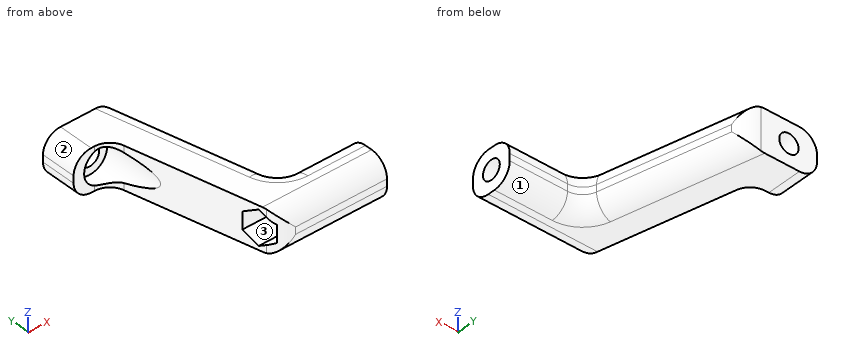
```python
from build123d import *

# Parameters (mm, degrees)
F1_DEPTH     = 12
F3_START     = -10
F2_R         = 2.75
F3_DEPTH     = 40.001
F4_DEPTH     = 50.001
F5_R         = 2.75
F6_DEPTH     = 55.001
F7_START     = -6
F5_R_2       = 5
F7_DEPTH     = 49.001
F8_T1_DEPTH  = 12
F8_T6_DEPTH  = 11.4445693846
F8_S7_R      = 5
F8_T8_DEPTH  = 8
F8_T12_DEPTH = 11.4445693846
F8_S13_R     = 5
F8_T14_DEPTH = 8
F8_T15_DEPTH = 55
F8_T17_DEPTH = 35
F8_T19_DEPTH = 28.9335864126
F8_T21_DEPTH = 32.0542901591
F8_T23_DEPTH = 52.5380765975
F8_T26_ANGLE = 77.4711922908
F8_T28_ANGLE = 77.4711922908


# Not quite as in the source:
# - a fillet or chamfer that OpenCascade refuses, or shapes differently, is made with other operations: its cross-section is extruded or revolved along the edge and cut away or added


with BuildPart() as f1:
    # F0 (on Top) → F1 (new body)
    with BuildSketch(Plane.XY):
        Polygon((-5.2704296331, 25.1133128916), (-25.2704296331, 25.1133128916), (-25.2704296331, 15.1133128916), (-15.2704296331, 15.1133128916), (-5.2704296331, -29.8866871084), (24.7295703669, -29.8866871084), (24.7295703669, -17.8866871084), (4.2851259224, -17.8866871084), align=None)
    extrude(amount=F1_DEPTH)

    # F2 (on face) → F3 (cut)
    with BuildSketch(Plane.YZ.offset(24.7295703669).offset(F3_START)):
        Polygon((-19.6366871084, 3.5462613559), (-19.6366871084, 8.4537386441), (-23.8866871084, 10.9074772881), (-28.1366871084, 8.4537386441), (-28.1366871084, 3.5462613559), (-23.8866871084, 1.0925227119), align=None)
        with Locations((-23.8866871084, 6)):
            Circle(F2_R, mode=Mode.SUBTRACT)
    extrude(amount=-F3_DEPTH, mode=Mode.SUBTRACT)

    # F2 (on face) → F4 (cut, through all)
    with BuildSketch(Plane.YZ.offset(24.7295703669)):
        with Locations((-23.8866871084, 6)):
            Circle(F2_R)
    extrude(amount=-F4_DEPTH, mode=Mode.SUBTRACT)

    # F5 (on face) → F6 (cut, through all)
    with BuildSketch(Plane(origin=(0, 25.1133128916, 0), x_dir=(-1, 0, 0), z_dir=(0, 1, 0))):
        with Locations((17.2704296331, 6)):
            Circle(F5_R)
    extrude(amount=-F6_DEPTH, mode=Mode.SUBTRACT)

    # F5 (on face) → F7 (cut)
    with BuildSketch(Plane(origin=(0, 25.1133128916, 0), x_dir=(-1, 0, 0), z_dir=(0, 1, 0)).offset(F7_START)):
        with Locations((17.2704296331, 6)):
            Circle(F5_R_2)
        with Locations((17.2704296331, 6)):
            Circle(F5_R, mode=Mode.SUBTRACT)
    extrude(amount=-F7_DEPTH, mode=Mode.SUBTRACT)

    # F8: fillet of radius 5 on 13 edges, made by hand

    # F8_s2 → F8_t1 (join)
    with BuildSketch(Plane.XY):
        with BuildLine():
            ThreePointArc((3.4150486533, -13.9713393975), (5.1673469863, -16.7868961698), (8.2959839543, -17.8866871084))
            Line((8.2959839543, -17.8866871084), (4.2851259224, -17.8866871084))
            Line((4.2851259224, -17.8866871084), (3.4150486533, -13.9713393975))
        make_face()
    extrude(amount=F8_T1_DEPTH)


with BuildPart() as f8_tool4:
    # F8_s5 → F8_t6 (new body)
    with BuildSketch(Plane.XY):
        with BuildLine():
            ThreePointArc((-19.281287665, 15.1133128916), (-16.152650697, 14.013521953), (-14.400352364, 11.1979651807))
            Line((-14.400352364, 11.1979651807), (-15.2704296331, 15.1133128916))
            Line((-15.2704296331, 15.1133128916), (-19.281287665, 15.1133128916))
        make_face()
    extrude(amount=F8_T6_DEPTH)

    # F8_s7 → F8_t8 (cut, symmetric)
    with BuildSketch(Plane.XZ.offset(-13.2)):
        with Locations((-17.2704296331, 6)):
            Circle(F8_S7_R)
    extrude(amount=F8_T8_DEPTH, both=True, mode=Mode.SUBTRACT)


with BuildPart() as f1_1:
    add(f1.part)

    # F8_t3: union F8_tool4
    add(f8_tool4.part)


with BuildPart() as f8_tool10:
    # F8_s11 → F8_t12 (new body)
    with BuildSketch(Plane.XY.offset(0.5554306154)):
        with BuildLine():
            ThreePointArc((-19.281287665, 15.1133128916), (-16.152650697, 14.013521953), (-14.400352364, 11.1979651807))
            Line((-14.400352364, 11.1979651807), (-15.2704296331, 15.1133128916))
            Line((-15.2704296331, 15.1133128916), (-19.281287665, 15.1133128916))
        make_face()
    extrude(amount=F8_T12_DEPTH)

    # F8_s13 → F8_t14 (cut, symmetric)
    with BuildSketch(Plane.XZ.offset(-13.2)):
        with Locations((-17.2704296331, 6)):
            Circle(F8_S13_R)
    extrude(amount=F8_T14_DEPTH, both=True, mode=Mode.SUBTRACT)


with BuildPart() as f1_2:
    add(f1_1.part)

    # F8_t9: union F8_tool10
    add(f8_tool10.part)

    # F8_s16 → F8_t15 (cut)
    with BuildSketch(Plane.YZ.offset(-17.7704296331)):
        with BuildLine():
            ThreePointArc((-29.8866871084, 7), (-28.4222210144, 10.5355339059), (-24.8866871084, 12))
            Line((-24.8866871084, 12), (-29.8866871084, 12))
            Line((-29.8866871084, 12), (-29.8866871084, 7))
        make_face()
        with BuildLine():
            ThreePointArc((-29.8866871084, 5), (-28.4222210144, 1.4644660941), (-24.8866871084, 0))
            Line((-24.8866871084, 0), (-29.8866871084, 0))
            Line((-29.8866871084, 0), (-29.8866871084, 5))
        make_face()
    extrude(amount=F8_T15_DEPTH, mode=Mode.SUBTRACT)

    # F8_s18 → F8_t17 (cut)
    with BuildSketch(Plane.XZ.offset(-37.6133128916)):
        with BuildLine():
            ThreePointArc((-25.2704296331, 7), (-23.8059635391, 10.5355339059), (-20.2704296331, 12))
            Line((-20.2704296331, 12), (-25.2704296331, 12))
            Line((-25.2704296331, 12), (-25.2704296331, 7))
        make_face()
        with BuildLine():
            ThreePointArc((-25.2704296331, 5), (-23.8059635391, 1.4644660941), (-20.2704296331, 0))
            Line((-20.2704296331, 0), (-25.2704296331, 0))
            Line((-25.2704296331, 0), (-25.2704296331, 5))
        make_face()
    extrude(amount=F8_T17_DEPTH, mode=Mode.SUBTRACT)

    # F8_s20 → F8_t19 (cut)
    with BuildSketch(Plane.YZ.offset(8.2959839543)):
        with BuildLine():
            ThreePointArc((-17.8866871084, 7), (-19.3511532025, 10.5355339059), (-22.8866871084, 12))
            Line((-22.8866871084, 12), (-17.8866871084, 12))
            Line((-17.8866871084, 12), (-17.8866871084, 7))
        make_face()
        with BuildLine():
            ThreePointArc((-17.8866871084, 5), (-19.3511532025, 1.4644660941), (-22.8866871084, 0))
            Line((-22.8866871084, 0), (-17.8866871084, 0))
            Line((-17.8866871084, 0), (-17.8866871084, 5))
        make_face()
    extrude(amount=F8_T19_DEPTH, mode=Mode.SUBTRACT)

    # F8_s22 → F8_t21 (cut)
    with BuildSketch(Plane.XY.offset(-10.0271450796)):
        with BuildLine():
            ThreePointArc((-6.1405069022, -25.9713393975), (-4.3882085693, -28.7868961698), (-1.2595716013, -29.8866871084))
            Line((-1.2595716013, -29.8866871084), (-5.2704296331, -29.8866871084))
            Line((-5.2704296331, -29.8866871084), (-6.1405069022, -25.9713393975))
        make_face()
        with BuildLine():
            ThreePointArc((-9.281287665, 25.1133128916), (-6.152650697, 24.013521953), (-4.400352364, 21.1979651807))
            Line((-4.400352364, 21.1979651807), (-5.2704296331, 25.1133128916))
            Line((-5.2704296331, 25.1133128916), (-9.281287665, 25.1133128916))
        make_face()
    extrude(amount=F8_T21_DEPTH, mode=Mode.SUBTRACT)

    # F8_s24 → F8_t23 (cut)
    with BuildSketch(Plane(origin=(3.1193447502, -14.037051376, 0), x_dir=(0, 0, 1), z_dir=(-0.2169304578, 0.9761870602, 0))):
        with BuildLine():
            ThreePointArc((0, -4.6970827466), (1.4644660941, -1.1615488406), (5, 0.3029172534))
            Line((5, 0.3029172534), (0, 0.3029172534))
            Line((0, 0.3029172534), (0, -4.6970827466))
        make_face()
        with BuildLine():
            ThreePointArc((12, -4.6970827466), (10.5355339059, -1.1615488406), (7, 0.3029172534))
            Line((7, 0.3029172534), (12, 0.3029172534))
            Line((12, 0.3029172534), (12, -4.6970827466))
        make_face()
    extrude(amount=F8_T23_DEPTH, mode=Mode.SUBTRACT)

    # F8_s25 → F8_t26 (revolve, cut)
    with BuildSketch(Plane(origin=(3.1193447502, -14.037051376, 0), x_dir=(0, 0, 1), z_dir=(-0.2169304578, 0.9761870602, 0))):
        with BuildLine():
            ThreePointArc((7, 0.3029172534), (10.5355339059, -1.1615488406), (12, -4.6970827466))
            Line((12, -4.6970827466), (12, 0.3029172534))
            Line((12, 0.3029172534), (7, 0.3029172534))
        make_face()
    revolve(axis=Axis((8.2959839543, -12.8866871084, 12), (0, 0, 1)), revolution_arc=F8_T26_ANGLE, mode=Mode.SUBTRACT)

    # F8_s27 → F8_t28 (revolve, cut)
    with BuildSketch(Plane(origin=(3.1193447502, -14.037051376, 0), x_dir=(0, 0, 1), z_dir=(-0.2169304578, 0.9761870602, 0))):
        with BuildLine():
            ThreePointArc((5, 0.3029172534), (1.4644660941, -1.1615488406), (0, -4.6970827466))
            Line((0, -4.6970827466), (0, 0.3029172534))
            Line((0, 0.3029172534), (5, 0.3029172534))
        make_face()
    revolve(axis=Axis((8.2959839543, -12.8866871084, 0), (0, 0, 1)), revolution_arc=F8_T28_ANGLE, mode=Mode.SUBTRACT)


solid = f1_2.part
```
CAD build for the part. Positions are in the model's coordinates, mm. Face numbers are marked on the shaded views. Round coordinates to 2 decimals unless told otherwise and drop trailing zeros. Loops run counter-clockwise (first coordinate to the right, second up) from the corner with the lowest first, then second, coordinate; pieces in that order, holes last. Notation, with made-up numbers: (9, -28) - (68, -28) arc R17 ccw to (68, 0) - close; hole circle Ø11 at (85, 35.5). An arc over 180 degrees is marked (long way). Return JSON: item names as keys, results as strings. Group by question number.
Q1. Two-plate mould, pull along Z, no slides. Class the marked faces 1, 2 and 3: +Z half, -Z half, draft (parallel to the pull), parting line (faces both ways), or undercut.
Q2. Drill centre lines: line 1 along Y through (x, z) = (-15, 3.5); line 2 along Z through (x, y) = (11.5, -26); line 3 along Y through (x, z) = (9, 9.25). Where is each one in solid material? Low to high. Write a range as [from, to].
Q3. Band-saw the part on B-B on x = 20. Give the cut face in (y, z).
Q4. Band-saw the part on A-A on z = 6. Give the cut face in (x, y), plus the area to 3 significant figures.
Q5. Flat gauge pins, fed straight in: pin 1 Ø3 at (y, z) = (-5.5, 2) entering from +X; pin 2 Ø2 at (y, z) = (-2, 5) entering from -X; pin 3 Ø1.6 at (x, z) = (17.5, 6) entering from +Y. Where does each tip first touch, or does it go through?
Solutions:
{
 "1": {"face 1": "-Z half", "face 2": "+Z half", "face 3": "undercut"},
 "2": {"line 1": "y = [19.11, 25.11]", "line 2": "z = [0.13, 2.31], [9.69, 11.87]", "line 3": "y = [-29.35, -26.76], [-21.02, -18.42]"},
 "3": {"outline": "(-29.89, 5) arc R5 ccw to (-24.89, 0) - (-22.89, 0) arc R5 ccw to (-17.89, 5) - (-17.89, 7) arc R5 ccw to (-22.89, 12) - (-24.89, 12) arc R5 ccw to (-29.89, 7) - close; hole circle Ø5.5 at (-23.89, 6)"},
 "4": {"outline": "(-25.27, 15.11) - (-22.27, 15.11) - (-22.27, 19.11) - (-20.02, 19.11) - (-20.02, 25.11) - (-25.27, 25.11) - close; (-14.52, 19.11) - (-12.27, 19.11) - (-12.27, 1.61) - (-7.55, -19.64) - (14.73, -19.64) - (14.73, -21.14) - (24.73, -21.14) - (24.73, -17.89) - (8.3, -17.89) arc R5 cw to (3.42, -13.97) - (-4.4, 21.2) arc R5 ccw to (-9.28, 25.11) - (-14.52, 25.11) - close; (-5.06, -28.14) arc R5 ccw to (-1.26, -29.89) - (24.73, -29.89) - (24.73, -26.64) - (14.73, -26.64) - (14.73, -28.14) - close", "area": "658 mm^2"},
 "5": {"pin 1": "stops at x = 1.39", "pin 2": "stops at x = -11.69", "pin 3": "stops at y = -17.89"}
}
